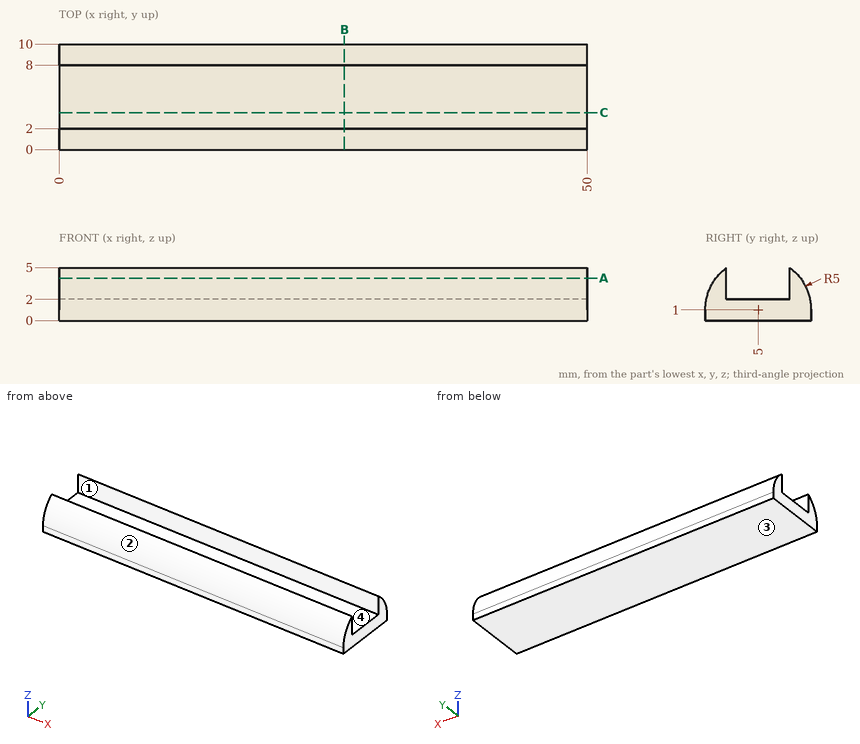
Check sheet for the drawn part. Datum: minimum x, y, z corner. Units: mm. Coordinates: 2 decimals unless noted, no trailing zeros. Write each loop counter-clockwise with the first axis right and the second up, starting at its lowest first coordinate (ties: lowest second). Pieces come first, ordered by that corner, then holes. Notation, with made-up numbers: (88.25, -31) - (138.25, -31) arc R30 cw to (138.25, -8) - close; hole circle Ø8 at (24.25, 7.5). An arc over 180 degrees is marked (long way). Answer as a JSON object with one key per item and string values.
(1) Mould release check, pull along Y, two halves, no side actions. Record for the marked faces 1, 2, 3 and 4: pulls with the +Y half, pulls with the -Y half, needs draft (parallel to the pull), parting line crosses it, or undercut.
Report:
{"face 1": "undercut", "face 2": "pulls with the -Y half", "face 3": "needs draft", "face 4": "undercut"}
(2) Cross-section at C-C on y = 3.5. Record the cut outline in (x, z).
Report:
{"outline": "(0, 0) - (50, 0) - (50, 2) - (0, 2) - close"}
(3) Cross-section at A-A on z = 4. Record the cut outline in (x, y), plus the area to 3 significant figures.
Report:
{"outline": "(0, 1) - (50, 1) - (50, 2) - (0, 2) - close; (0, 8) - (50, 8) - (50, 9) - (0, 9) - close", "area": "100 mm^2"}
(4) Gauge pin test, flat ends, axial feed: pin 1 Ø3 at (x, y) = (21.5, 1.5) entering from -Z; pin 2 Ø1 at (x, z) = (27, 4.5) entering from -Y; pin 3 Ø0.9 at (x, z) = (21.5, 4) entering from -Y; pin 4 Ø5 at (x, y) = (14, 6) entering from +Z. Record the tip position at first contact, or that the pin passes through.
Report:
{"pin 1": "z = 0", "pin 2": "y = 1", "pin 3": "y = 0.7", "pin 4": "z = 5"}
(5) Thickness scan on line 1 along Z through (x, y) = (4.5, 3.5); line 2 along Y through (x, z) = (8.5, 3.6); line 3 along Y through (x, z) = (33, 3.35). Record the ranges inside material, lowest first.
Report:
{"line 1": "0 to 2", "line 2": "0.73 to 2, 8 to 9.27", "line 3": "0.59 to 2, 8 to 9.41"}
(6) Cross-section at B-B on x = 27. Record the cut outline in (y, z).
Report:
{"outline": "(0, 0) - (10, 0) - (10, 1) arc R5 ccw to (8, 5) - (8, 2) - (2, 2) - (2, 5) arc R5 ccw to (0, 1) - close"}
